The figure shows three views and two pictorial views of one solid part (mm, origin at its lowest corner). Answer the questions. Coordinates: 2 decimals unless noted, no trailing zeros. Write each loop counter-clockwise with the first axis right and the second up, starting at its lowest first coordinate (ties: lowest second). Pieces come first, ordered by that corner, then holes.
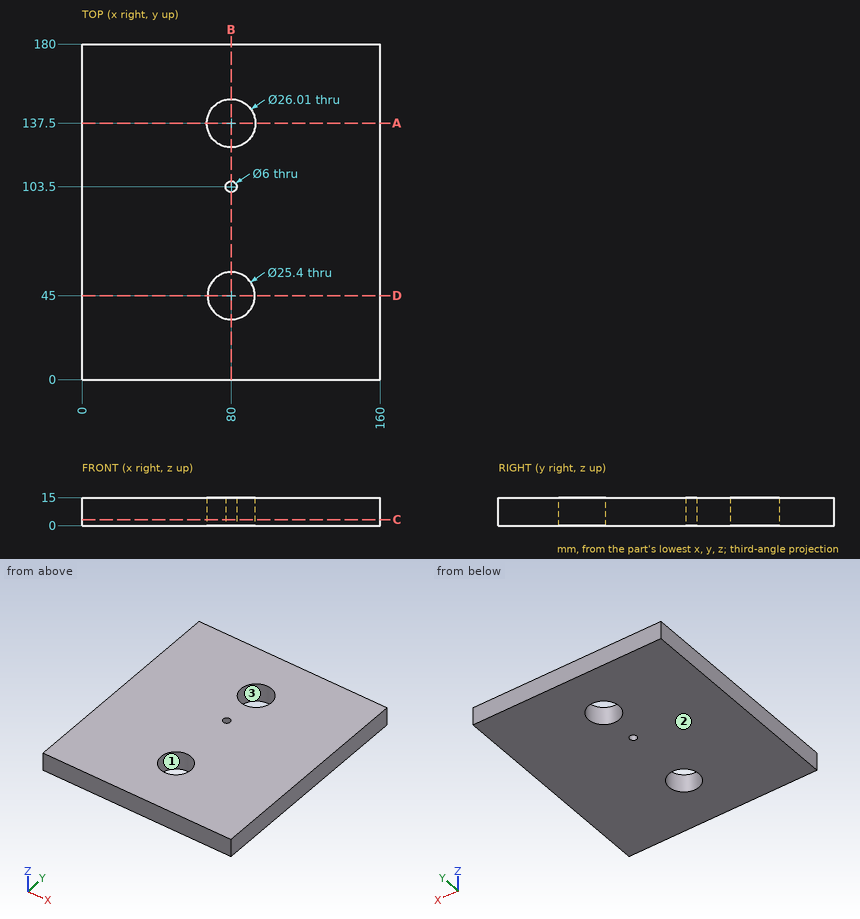
Q1. The part is cut by section D-D, the plane y = 45. Write down the section's boundary in (x, z), then the cut area to 3 significant figures.
Answers below:
outline: (0, 0) - (67.3, 0) - (67.3, 15) - (0, 15) - close; (92.7, 0) - (160, 0) - (160, 15) - (92.7, 15) - close
area: 2,020 mm2
Q2. Find the intervals of material crossed by probe 1 along Y at (x, z) = (80, 9) (3 decimals); probe 2 along Y at (x, z) = (83.5, 4); probe 3 along X at (y, z) = (104, 3), in increasing order.
Answers below:
probe 1: y = 0 to 32.3, 57.7 to 100.5, 106.5 to 124.495, 150.505 to 180
probe 2: y = 0 to 32.79, 57.21 to 124.97, 150.03 to 180
probe 3: x = 0 to 77.04, 82.96 to 160
Q3. The part is cut by section C-C, the plane z = 3.25. Write down the section's boundary in (x, y) (3 decimals), then the cut area to 3 significant figures.
Answers below:
outline: (0, 0) - (160, 0) - (160, 180) - (0, 180) - close; hole circle Ø26.01 at (80, 137.5); hole circle Ø25.4 at (80, 45); hole circle Ø6 at (80, 103.5)
area: 27,700 mm2
Q4. Determine the mould class of the marked faces 1, 2 and 3 for opening direction X: released by +X, released by -X, zero draft, split by the parting line, or undercut.
Answers below:
face 1: undercut
face 2: zero draft
face 3: undercut
Q5. The part is cut by section A-A, the plane y = 137.5. Write down the section's boundary in (x, z) (3 decimals).
Answers below:
outline: (0, 0) - (66.995, 0) - (66.995, 15) - (0, 15) - close; (93.005, 0) - (160, 0) - (160, 15) - (93.005, 15) - close
Q6. Given pin 1 (1 mm diameter, centred on x = 80.5, y = 115, fed in from -Z); pin 2 (15 mm diameter, centred on x = 80, y = 45, fed in from -Z), each flat-ended and moving along its own axis, determine where each tip first touches the part or whether it passes through.
Answers below:
pin 1: stops at z = 0
pin 2: passes through
Q7. The part is cut by section B-B, the plane x = 80. Write down the section's boundary in (y, z) (3 decimals).
Answers below:
outline: (0, 0) - (32.3, 0) - (32.3, 15) - (0, 15) - close; (57.7, 0) - (100.5, 0) - (100.5, 15) - (57.7, 15) - close; (106.5, 0) - (124.495, 0) - (124.495, 15) - (106.5, 15) - close; (150.505, 0) - (180, 0) - (180, 15) - (150.505, 15) - close
